Input: part model. Units: mm. Frame: model coordinates. Round coordinates to 2 decimals unless told otherwise and drop trailing zeros. Order: outer loops, then holes, each group sorted by start corner. A loop starts at its lowest first (then second) coordinate and runs counter-clockwise, first axis right, second up. Notation, with made-up numbers: (14, 38.5) - (64, 38.5) arc R25 ccw to (64, 65.5) - close; hole circle Ø1 at (1, 76.25). An arc over 180 degrees is marked (long way). One line per item, written item: value. Start each with the question number.
Solid Edge part; units mm, degrees
sketch "Sketch1" plane through (0, 0, 0) normal (1, 0, 0) x (0, 1, 0)
  arc A0 (1.1755, 2.1608) -> (1.1755, -2.1608) centre (-0.225, 0) ccw
  arc A1 (1.1755, -2.1608) -> (1.7194, -2) centre (1.7194, -3) cw
  line L0 (1.7194, -2) -> (3.5791, -2)
  arc A2 (3.5791, -2) -> (4.0694, -0.5) centre (0, 0) ccw
  line L1 (4.0694, -0.5) -> (1.833, -0.5)
  arc A3 (1.833, -0.5) -> (1.833, 0.5) centre (0, 0) cw
  line L2 (1.833, 0.5) -> (4.0694, 0.5)
  arc A4 (4.0694, 0.5) -> (3.5791, 2) centre (0, 0) ccw
  line L3 (3.5791, 2) -> (1.7194, 2)
  arc A5 (1.7194, 2) -> (1.1755, 2.1608) centre (1.7194, 3) cw
extrude "Protrusion1" add sketch "Sketch1" along normal blind 0.4
sketch "Sketch2" plane through (0, 0, 0) normal (1, 0, 0) x (0, 1, 0)
  line L0 (4.8771, 2.1) -> (2.9343, 2.1)
  line L1 (2.9343, 2.1) -> (2.9343, 2)
  arc A0 (2.9343, 2) -> (3.8808, 1.3226) centre (2.9343, 1) cw
  arc A1 (3.8808, 1.3226) -> (4.0694, 0.5) centre (0, 0) cw
  line L2 (4.0694, 0.5) -> (4.0694, -0.5)
  arc A2 (4.0694, -0.5) -> (3.8808, -1.3226) centre (0, 0) cw
  arc A3 (3.8808, -1.3226) -> (2.9343, -2) centre (2.9343, -1) cw
  line L3 (2.9343, -2) -> (2.9343, -2.1)
  line L4 (2.9343, -2.1) -> (4.8771, -2.1)
  arc A4 (4.8771, -2.1) -> (4.8771, 2.1) centre (0, 0) ccw
extrude "Extrusionsausschnitt_1" cut sketch "Sketch2" along normal blind 0.4
sketch "Sketch3" plane through (0, 0, 0) normal (1, 0, 0) x (0, 1, 0)
  arc A0 (3.4512, 0.5) -> (2.4512, 0.5) centre (2.9512, 0.5) ccw
  line L0 (2.4512, 0.5) -> (2.4512, -0.5)
  arc A1 (2.4512, -0.5) -> (3.4512, -0.5) centre (2.9512, -0.5) ccw
  line L1 (3.4512, -0.5) -> (3.4512, 0.5)
extrude "Extrusionsausschnitt_2" cut sketch "Sketch3" along normal blind 0.4
properties part number "Retaining ring DIN 471 4x0.4 36000.004.001(High)"
1. Section A-A (z = 1.4). Return the cut outline in (x, y), then the cut area to 3 significant figures.
2. Section D-D (z = -0.1). Return the cut outline in (x, y), then the cut area to 3 significant figures.
3. Pull-direction query (Z, two-part tool) for faces 1 (the face through (0.2, -1.9, -0.08)), 2 (the face through (0.2, -2.8, -0.1)), 3 (the face through (0, 2, 1)); classes: released by +Z, released by -Z, zero draft, split by the parting line, or undercut.
4. Pin query (flat end, axial travel): pin 1 (3 mm diameter, centred on y = -0.5, z = 1.5, fed in from +X). Return the tip coordinate at first contact, or that it passes through.
5. Line query: line 1 (Y direction, x = 0.25, z = -0.65); line 2 (Z direction, x = 0.1, y = 0); line 3 (Z direction, x = 0.3, y = 0.5). Output: solid intervals per line, ascending. Write a range as from..to.
6. Section B-B (y = -0.25). Return the cut outline in (x, z).
Solved:
1. outline: (0, -2.39) - (0.4, -2.39) - (0.4, -1.28) - (0, -1.28) - close; (0, 1.28) - (0.4, 1.28) - (0.4, 3.85) - (0, 3.85) - close
1. area: 1.47 mm²
2. outline: (0, -2.8) - (0.4, -2.8) - (0.4, -1.9) - (0, -1.9) - close
2. area: 0.360 mm²
3. face 1: undercut
3. face 2: split by the parting line
3. face 3: zero draft
4. pin 1: stops at x = 0.4
5. line 1: y = -2.72..-1.79, 1.79..2.47, 3.43..4.05
5. line 2: z = -2.57..-1.9, 1.9..2.57
5. line 3: z = -2.47..-1.83, 1.83..2.47
6. outline: (0, -2.57) - (0.4, -2.57) - (0.4, -1.88) - (0, -1.88) - close; (0, 1.88) - (0.4, 1.88) - (0.4, 2.57) - (0, 2.57) - close
